from build123d import *

# Parameters (mm, degrees)
SKETCH1_W                 = 69.85
SKETCH1_H                 = 38.1
BOSS_EXTRUDE1_DEPTH       = 6.35
F_6_CLEARANCE_HOLE1_D     = 3.7973
F_6_CLEARANCE_HOLE1_DEPTH = 25.4
F_6_CLEARANCE_HOLE1_TIP   = 1.140824014
FILLET1_R                 = 6.35


with BuildPart() as part:
    # Sketch1 → Boss-Extrude1 (new body)
    with BuildSketch(Plane(origin=(0, 0, 0), x_dir=(1, 0, 0), z_dir=(0, 1, 0))):
        Rectangle(SKETCH1_W, SKETCH1_H)
    extrude(amount=BOSS_EXTRUDE1_DEPTH)

    # #6 Clearance Hole1
    with Locations(Plane.XZ):
        with Locations((-25.4, 9.525), (25.4, -9.525), (-25.4, -9.525), (25.4, 9.525)):
            Hole(F_6_CLEARANCE_HOLE1_D / 2, depth=F_6_CLEARANCE_HOLE1_DEPTH)
            with Locations((0, 0, -(F_6_CLEARANCE_HOLE1_DEPTH + F_6_CLEARANCE_HOLE1_TIP / 2))):  # 118° drill point
                Cone(0, F_6_CLEARANCE_HOLE1_D / 2, F_6_CLEARANCE_HOLE1_TIP, mode=Mode.SUBTRACT)

    # Fillet1
    fillet1_edges = [part.edges().sort_by_distance(p)[0] for p in [
        (-34.925, 3.175, -19.05),
        (34.925, 3.175, -19.05),
        (34.925, 3.175, 19.05),
        (-34.925, 3.175, 19.05),
    ]]
    fillet(fillet1_edges, radius=FILLET1_R)


solid = part.part
Source: CAD feature listing. Evaluate the final solid. Frame: model axes, mm. Give positions to 0.01 mm unless a question says otherwise; leave off trailing zeros. Write each loop counter-clockwise with the first axis right and the second up, starting at its lowest first coordinate (ties: lowest second). Pieces come first, ordered by that corner, then holes. Notation, with made-up numbers: M 2.25,23.25 L 60.25,23.25 A16 cw 60.25,46.25 Z; hole C 76,81.25 d5. An arc over 180 degrees is marked long. Answer as a JSON object with one key per item and string values.
Q1. Mould query, pull axis X, two halves, no side actions, for faces 1 (the face through (-23.503, 3.219, 9.608)), 2 (the face through (-33.114, 3.219, 17.14)), 3 (the face through (0, 3, -19.05)). Classes: +X half, -X half, draft (parallel to the pull), parting line (faces both ways), or undercut.
Geometry check:
{"face 1": "undercut", "face 2": "-X half", "face 3": "draft"}
Q2. Ray query, line 1 along Z through (x, y) = (25.4, 3.5); line 2 along X through (y, z) = (4, 8.5) (3 decimals); line 3 along X through (y, z) = (2, 9) (3 decimals). Return the intervals inside material, ascending.
Geometry check:
{"line 1": "z = -19.05 to -11.42, -7.63 to 7.63, 11.42 to 19.05", "line 2": "x = -34.925 to -26.998, -23.802 to 23.802, 26.998 to 34.925", "line 3": "x = -34.925 to -27.225, -23.575 to 23.575, 27.225 to 34.925"}
Q3. Cut plane B-B, the plane z = -10.5. Return the cut outline in (x, y) (3 decimals).
Geometry check:
{"outline": "M -34.925,0 L -27.029,0 L -27.029,6.35 L -34.925,6.35 Z; M -23.771,0 L 23.771,0 L 23.771,6.35 L -23.771,6.35 Z; M 27.029,0 L 34.925,0 L 34.925,6.35 L 27.029,6.35 Z"}
Q4. Cut plane A-A, the plane x = 25.4. Return the cut outline in (y, z).
Geometry check:
{"outline": "M 0,-19.05 L 6.35,-19.05 L 6.35,-11.42 L 0,-11.42 Z; M 0,-7.63 L 6.35,-7.63 L 6.35,7.63 L 0,7.63 Z; M 0,11.42 L 6.35,11.42 L 6.35,19.05 L 0,19.05 Z"}
Q5. Cut plane C-C, the plane y = 4.5. Return the cut outline in (x, z) (3 decimals), then the cut area to 3 significant figures.
Geometry check:
{"outline": "M -34.925,-12.7 A6.35 ccw -28.575,-19.05 L 28.575,-19.05 A6.35 ccw 34.925,-12.7 L 34.925,12.7 A6.35 ccw 28.575,19.05 L -28.575,19.05 A6.35 ccw -34.925,12.7 Z; hole C -25.4,-9.525 d3.797; hole C -25.4,9.525 d3.797; hole C 25.4,-9.525 d3.797; hole C 25.4,9.525 d3.797", "area": "2,580 mm^2"}
